```python
from build123d import *

# Parameters (mm, degrees)
F0_R      = 38
F1_DEPTH  = 10
F4_DEPTH  = 4.5
F5_R      = 1
F6_COUNT  = 16
F7_R      = 12.5
F8_DEPTH  = 98
F9_DEPTH  = 14
F11_DEPTH = 26
F13_R     = 38
F14_DEPTH = 5
F15_SIZE  = 2


with BuildPart() as f1:
    # F0 (on Front) → F1 (new body)
    with BuildSketch(Plane.XZ):
        Circle(F0_R)
    extrude(amount=F1_DEPTH)

    # F3 (on mid) → F4 (join, symmetric)
    with BuildSketch(Plane.XZ.offset(5)):
        with BuildLine():
            Line((-47.9583152331, -2), (-37.7888872554, -4))
            Line((-37.7888872554, -4), (-37.7888872554, 4))
            Line((-37.7888872554, 4), (-47.9583152331, 2))
            ThreePointArc((-47.9583152331, 2), (-48, 0), (-47.9583152331, -2))
        make_face()
    extrude(amount=F4_DEPTH, both=True)

    # F5
    f5_edges = [f1.edges().sort_by_distance(p)[0] for p in [
        (-47.958315, -5, -2),
        (-47.958315, -5, 2),
    ]]
    fillet(f5_edges, radius=F5_R)


with BuildPart() as f6_1:
    # F6: instance of F1
    add(f1.part.rotate(Axis((0, 0, 0), (0, -1, 0)), 1 * 360 / F6_COUNT))


with BuildPart() as f6_2:
    # F6: instance of F1
    add(f1.part.rotate(Axis((0, 0, 0), (0, -1, 0)), 2 * 360 / F6_COUNT))


with BuildPart() as f6_3:
    # F6: instance of F1
    add(f1.part.rotate(Axis((0, 0, 0), (0, -1, 0)), 3 * 360 / F6_COUNT))


with BuildPart() as f6_4:
    # F6: instance of F1
    add(f1.part.rotate(Axis((0, 0, 0), (0, -1, 0)), 4 * 360 / F6_COUNT))


with BuildPart() as f6_5:
    # F6: instance of F1
    add(f1.part.rotate(Axis((0, 0, 0), (0, -1, 0)), 5 * 360 / F6_COUNT))


with BuildPart() as f6_6:
    # F6: instance of F1
    add(f1.part.rotate(Axis((0, 0, 0), (0, -1, 0)), 6 * 360 / F6_COUNT))


with BuildPart() as f6_7:
    # F6: instance of F1
    add(f1.part.rotate(Axis((0, 0, 0), (0, -1, 0)), 7 * 360 / F6_COUNT))


with BuildPart() as f6_8:
    # F6: instance of F1
    add(f1.part.rotate(Axis((0, 0, 0), (0, -1, 0)), 8 * 360 / F6_COUNT))


with BuildPart() as f6_9:
    # F6: instance of F1
    add(f1.part.rotate(Axis((0, 0, 0), (0, -1, 0)), 9 * 360 / F6_COUNT))


with BuildPart() as f6_10:
    # F6: instance of F1
    add(f1.part.rotate(Axis((0, 0, 0), (0, -1, 0)), 10 * 360 / F6_COUNT))


with BuildPart() as f6_11:
    # F6: instance of F1
    add(f1.part.rotate(Axis((0, 0, 0), (0, -1, 0)), 11 * 360 / F6_COUNT))


with BuildPart() as f6_12:
    # F6: instance of F1
    add(f1.part.rotate(Axis((0, 0, 0), (0, -1, 0)), 12 * 360 / F6_COUNT))


with BuildPart() as f6_13:
    # F6: instance of F1
    add(f1.part.rotate(Axis((0, 0, 0), (0, -1, 0)), 13 * 360 / F6_COUNT))


with BuildPart() as f6_14:
    # F6: instance of F1
    add(f1.part.rotate(Axis((0, 0, 0), (0, -1, 0)), 14 * 360 / F6_COUNT))


with BuildPart() as f6_15:
    # F6: instance of F1
    add(f1.part.rotate(Axis((0, 0, 0), (0, -1, 0)), 15 * 360 / F6_COUNT))


with BuildPart() as f8:
    # F7 (on face) → F8 (new body)
    with BuildSketch(Plane.XZ.offset(10)):
        Circle(F7_R)
    extrude(amount=-F8_DEPTH)


with BuildPart() as f9:
    # F9 (new): a face of the model
    f9_faces = [f8.part.faces().sort_by_distance(p)[0] for p in [
        (0, -10, 0),
    ]]
    extrude(f9_faces, amount=F9_DEPTH)

    # F10 (on face) → F11 (join)
    with BuildSketch(Plane.XZ.offset(24)):
        Polygon((8.7402150444, 1.5656130559), (4.2253893698, 7.8095190592), (-3.4712406825, 8.1726979258), (-8.5539557005, 2.3816685616), (-7.1953676071, -5.2028058067), (-0.4185209468, -8.8694612846), (6.6734805227, -5.8572315112), align=None)
    extrude(amount=F11_DEPTH)


with BuildPart() as f1_1:
    add(f1.part)

    add(f6_1.part)  # F14 merges F6_1

    add(f6_2.part)  # F14 merges F6_2

    add(f6_3.part)  # F14 merges F6_3

    add(f6_4.part)  # F14 merges F6_4

    add(f6_5.part)  # F14 merges F6_5

    add(f6_6.part)  # F14 merges F6_6

    add(f6_7.part)  # F14 merges F6_7

    add(f6_8.part)  # F14 merges F6_8

    add(f6_9.part)  # F14 merges F6_9

    add(f6_10.part)  # F14 merges F6_10

    add(f6_11.part)  # F14 merges F6_11

    add(f6_12.part)  # F14 merges F6_12

    add(f6_13.part)  # F14 merges F6_13

    add(f6_14.part)  # F14 merges F6_14

    add(f6_15.part)  # F14 merges F6_15

    add(f8.part)  # F14 merges F8

    add(f9.part)  # F14 merges F9
    # F13 (on offset) → F14 (join, symmetric)
    with BuildSketch(Plane(origin=(0, 75, 0), x_dir=(-1, 0, 0), z_dir=(0, 1, 0))):
        Circle(F13_R)
    extrude(amount=F14_DEPTH, both=True)

    # F15
    f15_edges = [f1_1.edges().sort_by_distance(p)[0] for p in [
        (38, 80, 0),
        (38, 70, 0),
    ]]
    chamfer(f15_edges, length=F15_SIZE)


solid = f1_1.part
```
Build history of the part. All positions in model axes, mm. A direction names the side the tool comes from. Coordinates: 2 decimals unless noted, no trailing zeros. Order: outer loops, then holes, each group sorted by start corner. A loop starts at its lowest first (then second) coordinate and runs counter-clockwise, first axis right, second up.
Item 1: Saw through at A-A on y = 33. List the corners of the cut face in (x, z).
Filled in:
outline: circle Ø25 at (0, 0)
Item 2: Mould opens along X. For faces 6 (the cylindrical face through (-17.535, 75.042, -33.713)), 7 (the flat face through (-30, -9.5, -30)), 8 (the flat face through (-3.064, -5.063, 42.549)) say: released by +X, released by -X, zero draft, split by the parting line, or undercut.
Filled in:
face 6: split by the parting line
face 7: zero draft
face 8: undercut
Item 3: Drop flat-ended pins along their axis: pin 1 Ø3.5 at (x, z) = (-29, -30.5) entering from +Y; pin 2 Ø4 at (x, z) = (-36, 34) entering from -Y; pin 3 Ø10 at (y, z) = (-16.5, 35) entering from +X; pin 4 Ø10 at (x, z) = (-14.5, 37) entering from -Y. Give the stop position or say it passes through.
Filled in:
pin 1: stops at y = -0.5
pin 2: stops at y = -9.5
pin 3: passes through
pin 4: stops at y = -10
Item 4: Drill centre lines: L1, parallel to Y at x = 7.5, z = -27.5; L2, parallel to X at y = -1.5, z = -39; L3, parallel to X at y = -8.5, z = 30.5. Where is each one in solid material? Low to high.
Filled in:
L1: y = -10 to 0, 70 to 80
L2: x = -19.29 to -12.47, -3.76 to 3.76, 12.47 to 19.29
L3: x = -33.98 to -25.31, -22.67 to 22.67, 25.31 to 33.98
Item 5: Tool access for faces 1 (the flat face through (40.48, -5.06, -13.45)), 2 (the flat face through (-5.977, -36.818, 5.318)), 3 (the flat face through (-39, -9.5, -16)), 4 (the flat face through (3.078, -36.818, -7.384)), 5 (the flat face through (38.007, -5.063, -19.087)): list every direction of +Z, -Z, +X, -X, +Y, -Y with a clear straight run to the whole face (end or side of a thin tool).
Filled in:
face 1: +X, +Y, -Y
face 2: +Z, -X, -Y
face 3: -Z, -X, -Y
face 4: -Z, +X, -Y
face 5: +Y, -Y
